from build123d import *

# Parameters (mm, degrees)
SKETCH1_W           = 27.8
SKETCH1_H           = 15.9
BOSS_EXTRUDE1_DEPTH = 5.15
SKETCH4_R           = 1.55
CUT_EXTRUDE1_DEPTH  = 11.3
CUT_EXTRUDE2_DEPTH  = 0.6
SKETCH8_R           = 0.8
BOSS_EXTRUDE2_DEPTH = 0.25
LPATTERN1_COUNT     = 2
LPATTERN1_PITCH     = 6.5
BOSS_EXTRUDE3_DEPTH = 5
SKETCH10_W          = 4.75
SKETCH10_H          = 0.5
BOSS_EXTRUDE4_DEPTH = 6.35
CUT_EXTRUDE3_REACH  = 20.8
SKETCH11_R          = 0.8
BOSS_EXTRUDE5_DEPTH = 2.15
BOSS_EXTRUDE7_DEPTH = 2.25
FILLET1_R           = 2.8
FILLET2_R           = 1


with BuildPart() as part:
    # Sketch1 → Boss-Extrude1 (new body, symmetric)
    with BuildSketch(Plane(origin=(0, 0, 0), x_dir=(0, 0, -1), z_dir=(1, 0, 0))):
        Rectangle(SKETCH1_W, SKETCH1_H)
    extrude(amount=BOSS_EXTRUDE1_DEPTH, both=True)

    # Sketch4 → Cut-Extrude1 (cut, through all)
    with BuildSketch(Plane(origin=(5.15, 0, 0), x_dir=(0, 0, -1), z_dir=(1, 0, 0))):
        with Locations((11.1, 5.15)):
            Circle(SKETCH4_R)
        with BuildLine():
            Line((-11.325, -3.6), (-10.875, -3.6))
            ThreePointArc((-10.875, -3.6), (-9.325, -5.15), (-10.875, -6.7))
            Line((-10.875, -6.7), (-11.325, -6.7))
            ThreePointArc((-11.325, -6.7), (-12.875, -5.15), (-11.325, -3.6))
        make_face()
    extrude(amount=-CUT_EXTRUDE1_DEPTH, mode=Mode.SUBTRACT)

    # Sketch5 → Cut-Extrude2 (cut)
    with BuildSketch(Plane(origin=(5.15, 0, 0), x_dir=(0, 0, -1), z_dir=(1, 0, 0))):
        with BuildLine():
            Line((13.9, 2.35), (11.1, 2.35))
            ThreePointArc((11.1, 2.35), (9.120101013, 3.170101013), (8.3, 5.15))
            Line((8.3, 5.15), (8.3, 7.95))
            Line((8.3, 7.95), (13.9, 7.95))
            Line((13.9, 7.95), (13.9, 2.35))
        make_face()
        with BuildLine():
            Line((-13.9, -2.35), (-11.1, -2.35))
            ThreePointArc((-11.1, -2.35), (-9.120101013, -3.170101013), (-8.3, -5.15))
            Line((-8.3, -5.15), (-8.3, -7.95))
            Line((-8.3, -7.95), (-13.9, -7.95))
            Line((-13.9, -7.95), (-13.9, -2.35))
        make_face()
    extrude(amount=-CUT_EXTRUDE2_DEPTH, mode=Mode.SUBTRACT)

    # Sketch8 → Boss-Extrude2 (add, symmetric)
    with BuildSketch(Plane(origin=(0, 2.45, 0), x_dir=(1, 0, 0), z_dir=(0, 1, 0))):
        Polygon((-2.5, 13.9), (2.5, 13.9), (2.5, 17.55), (2.25, 17.55), (2.25, 23.9), (-2.25, 23.9), (-2.25, 17.55), (-2.5, 17.55), align=None)
        with Locations((0, 20.75)):
            Circle(SKETCH8_R, mode=Mode.SUBTRACT)
    boss_extrude2 = extrude(amount=BOSS_EXTRUDE2_DEPTH, both=True)

    # LPattern1: Boss-Extrude2 ×2
    with Locations(*[(0, -i * LPATTERN1_PITCH, 0) for i in range(1, LPATTERN1_COUNT)]):
        add(boss_extrude2)

    # Sketch9 → Boss-Extrude3 (add)
    with BuildSketch(Plane(origin=(2.5, 0, 0), x_dir=(0, 0, -1), z_dir=(1, 0, 0))):
        with BuildLine():
            Line((1.1, -7.95), (1.1, -9.85))
            ThreePointArc((1.1, -9.85), (1.392893219, -10.557106781), (2.1, -10.85))
            Line((2.1, -10.85), (4.75, -10.85))
            Line((4.75, -10.85), (4.75, -10.35))
            Line((4.75, -10.35), (2.1, -10.35))
            ThreePointArc((2.1, -10.35), (1.746446609, -10.203553391), (1.6, -9.85))
            Line((1.6, -9.85), (1.6, -7.95))
            Line((1.6, -7.95), (1.1, -7.95))
        make_face()
    extrude(amount=-BOSS_EXTRUDE3_DEPTH)

    # Sketch10 → Boss-Extrude4 (add)
    with BuildSketch(Plane(origin=(0, 0, -4.75), x_dir=(-1, 0, 0), z_dir=(0, 0, -1))):
        with Locations((0, -10.6)):
            Rectangle(SKETCH10_W, SKETCH10_H)
    extrude(amount=BOSS_EXTRUDE4_DEPTH)

    # Sketch11 → Cut-Extrude3 (cut, up to next)
    with BuildSketch(Plane.XZ.offset(10.85), mode=Mode.PRIVATE) as cut_extrude3_sk1:
        with Locations((0, -7.95)):
            Circle(SKETCH11_R)
    cut_extrude3_tool1 = extrude(cut_extrude3_sk1.sketch, amount=-CUT_EXTRUDE3_REACH, mode=Mode.PRIVATE) & part.part
    add(cut_extrude3_tool1.solids().sort_by_distance((0, -10.85, -7.95))[0], mode=Mode.SUBTRACT)

    # Sketch12 → Boss-Extrude5 (add, symmetric)
    with BuildSketch(Plane(origin=(0, 0, 0), x_dir=(0, 0, -1), z_dir=(1, 0, 0))):
        with BuildLine():
            Line((3.25, 7.95), (3.25, 9.05))
            ThreePointArc((3.25, 9.05), (3.030330086, 9.580330086), (2.5, 9.8))
            Line((2.5, 9.8), (-48.3, 9.8))
            Line((-48.3, 9.8), (-48.3, 9.3))
            Line((-48.3, 9.3), (2.5, 9.3))
            ThreePointArc((2.5, 9.3), (2.676776695, 9.226776695), (2.75, 9.05))
            Line((2.75, 9.05), (2.75, 7.95))
            Line((2.75, 7.95), (3.25, 7.95))
        make_face()
    extrude(amount=BOSS_EXTRUDE5_DEPTH, both=True)

    # Sketch13 → Boss-Extrude7 (add, symmetric)
    with BuildSketch(Plane(origin=(0, 0, 0), x_dir=(0, 0, -1), z_dir=(1, 0, 0))):
        with BuildLine():
            Line((-8.8, 8.85), (-8.8, 7.95))
            Line((-8.8, 7.95), (-7.8, 7.95))
            Line((-7.8, 7.95), (-7.8, 8.85))
            ThreePointArc((-7.8, 8.85), (-7.931801948, 9.168198052), (-8.25, 9.3))
            Line((-8.25, 9.3), (-8.35, 9.3))
            ThreePointArc((-8.35, 9.3), (-8.668198052, 9.168198052), (-8.8, 8.85))
        make_face()
    extrude(amount=BOSS_EXTRUDE7_DEPTH, both=True)

    # Fillet1
    fillet1_edges = [part.edges().sort_by_distance(p)[0] for p in [
        (-0.3, 7.95, -13.9),
        (-0.3, -7.95, 13.9),
        (0, -7.95, -13.9),
        (0, 7.95, 13.9),
    ]]
    fillet(fillet1_edges, radius=FILLET1_R)

    # Fillet2
    fillet2_edges = [part.edges().sort_by_distance(p)[0] for p in [
        (2.375, -10.6, -11.1),
        (-2.375, -10.6, -11.1),
        (2.25, -4.05, -23.9),
        (-2.25, -4.05, -23.9),
        (-2.25, 2.45, -23.9),
        (2.25, 2.45, -23.9),
    ]]
    fillet(fillet2_edges, radius=FILLET2_R)


solid = part.part
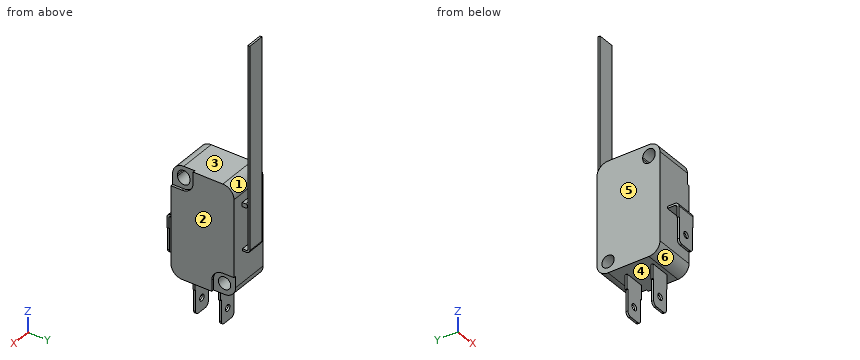
Work out the finished part from the listing and answer in its coordinate system (mm). Face numbers are marked on the shaded views. A direction names the side the tool comes from. Give positions to 0.01 mm unless a question says otherwise; leave off trailing zeros. Order: outer loops, then holes, each group sorted by start corner. A loop starts at its lowest first (then second) coordinate and runs counter-clockwise, first axis right, second up. Notation, with made-up numbers: (11.5, 50.5) -> (19.5, 50.5) arc R10 ccw to (19.5, 58.5) -> close; hole circle Ø2 at (17.5, -37.75). An arc over 180 degrees is marked (long way). One line per item, written item: value.
Item 1: Straight lines are drawn through the part: probe 1 along Z at (x, y) = (0, -10.55); probe 2 along Y at (x, z) = (1.5, -5.5); probe 3 along Z at (x, y) = (0, 2.35). For each, find the intervals that lie inside material, in ascending order.
Answer sheet:
probe 1: -11.1 to -8.75, -7.15 to -1.39
probe 2: -10.85 to -10.35, -7.95 to 7.95
probe 3: -23.9 to -21.55, -19.95 to 13.9
Item 2: Flat-ended cylindrical pins translate along their axes: P1, Ø0.6, axis at x = -0.5, y = -8.5, coming from the +Z side; P2, Ø6, axis at x = 1.5, y = 4.5, coming from the +Z side; P3, Ø3, axis at y = -6, z = 11.5, coming from the +X side; P4, Ø1.3, axis at x = 0, z = -20.75, coming from the +Y side. Find the tip coordinate at first contact, or state that the pin passes through.
Answer sheet:
P1: z = -1.1
P2: z = 13.9
P3: x = 4.55
P4: through
Item 3: Find section B-B, the plane z = -20.75. Give the vertices of the cut face in (x, y).
Answer sheet:
outline: (-2.25, -4.3) -> (-0.8, -4.3) -> (-0.8, -3.8) -> (-2.25, -3.8) -> close; (-2.25, 2.2) -> (-0.8, 2.2) -> (-0.8, 2.7) -> (-2.25, 2.7) -> close; (0.8, -4.3) -> (2.25, -4.3) -> (2.25, -3.8) -> (0.8, -3.8) -> close; (0.8, 2.2) -> (2.25, 2.2) -> (2.25, 2.7) -> (0.8, 2.7) -> close
Item 4: Find section A-A, the plane z = 5. Give the vertices of the cut face in (x, y).
Answer sheet:
outline: (-5.15, -7.95) -> (5.15, -7.95) -> (5.15, 7.95) -> (-5.15, 7.95) -> close; (-2.15, 9.3) -> (2.15, 9.3) -> (2.15, 9.8) -> (-2.15, 9.8) -> close
Item 5: Determine the mould class of the marked faces 4, 5 and 6 for opening direction Y: released by +Y, released by -Y, zero draft, split by the parting line, or undercut.
Answer sheet:
face 4: undercut
face 5: zero draft
face 6: released by -Y
Item 6: Find section C-C, the plane y = 4.5. Give the vertices of the cut face in (x, z).
Answer sheet:
outline: (-5.15, -13.9) -> (4.55, -13.9) -> (4.55, -12.51) -> (-5.15, -12.51) -> close; (-5.15, -9.69) -> (4.55, -9.69) -> (4.55, -8.38) -> (5.15, -8.38) -> (5.15, 13.9) -> (-5.15, 13.9) -> close
Item 7: A tool of negligible diameter and unlimited length cuts with its end or side. For the marked faces 1, 2 and 3, from which of +Z, -Z, +X, -X, +Y, -Y can it reach the whole face along a straight path? Write none if from no direction.
Answer sheet:
face 1: +Z, +X, -X
face 2: +Z, -Z, +X, +Y, -Y
face 3: +Z, +X, -X, -Y
Item 8: Find section D-D, the plane x = 0. State how many separate pieces and enclosed holes the cut face has, plus the area to 3 significant figures.
Answer sheet:
separate pieces: 4
enclosed holes: 3
area: 460 mm²
